from build123d import *

# Parameters (mm, degrees)
SKETCH_1_R      = 1.6
SKETCH_1_R_2    = 1.7
EXTRUDE_1_DEPTH = 3


with BuildPart() as part:
    # 草图1 → 凸台-拉伸1 (new body)
    with BuildSketch(Plane.XY):
        with BuildLine():
            Line((-53.850242828, 4), (171.149757172, 4))
            ThreePointArc((171.149757172, 4), (175.149757172, 0), (171.149757172, -4))
            Line((171.149757172, -4), (-53.850242828, -4))
            ThreePointArc((-53.850242828, -4), (-57.850242828, 0), (-53.850242828, 4))
        make_face()
        with Locations((-53.850242828, 0)):
            Circle(SKETCH_1_R, mode=Mode.SUBTRACT)
        with Locations((171.149757172, 0)):
            Circle(SKETCH_1_R_2, mode=Mode.SUBTRACT)
        with Locations((151.149757172, 0)):
            Circle(SKETCH_1_R_2, mode=Mode.SUBTRACT)
        with Locations((-33.850242828, 0)):
            Circle(SKETCH_1_R_2, mode=Mode.SUBTRACT)
    extrude(amount=EXTRUDE_1_DEPTH)


solid = part.part
For this review, take the finished solid that the model builds, in its own axes (mm). Give positions to 0.01 mm unless a question says otherwise; leave off trailing zeros. Order: outer loops, then holes, each group sorted by start corner. A loop starts at its lowest first (then second) coordinate and runs counter-clockwise, first axis right, second up. Notation, with made-up numbers: M -39,-2 L -15,-2 A27 ccw -15,16 Z; hole C -15.5,-14 d4. An arc over 180 degrees is marked long. Answer in a Markdown table with one row per item. Add a question column.
(1) Wall thickness on probe 1 along X at (y, z) = (1, 2.35); probe 2 along X at (y, z) = (1.25, 2.55); probe 3 along X at (y, z) = (3, 1.8): over which ranges is each line inside the solid? List them lowest first. Write a range as [from, to].
(2) Consider section A-A on y = 0. State the section outline as (x, z) points.
(3) For pin 1 (3 mm diameter, centred on x = 35.5, y = -2, fed in from -Z); pin 2 (2.5 mm diameter, centred on x = 171.15, y = 0, fed in from +Z), all flat-tipped, find the tip position at first contact; note any pin that passes through.
(4) Consider section B-B on z = 2.05. State the section outline as (x, y) points.
Evaluation:
| question | item | result |
|---|---|---|
| 1 | probe 1 | x = [-57.72, -55.1], [-52.6, -35.23], [-32.48, 149.77], [152.52, 169.77], [172.52, 175.02] |
| 1 | probe 2 | x = [-57.65, -54.85], [-52.85, -35], [-32.7, 150], [152.3, 170], [172.3, 174.95] |
| 1 | probe 3 | x = [-56.5, 173.8] |
| 2 | outline | M -57.85,0 L -55.45,0 L -55.45,3 L -57.85,3 Z; M -52.25,0 L -35.55,0 L -35.55,3 L -52.25,3 Z; M -32.15,0 L 149.45,0 L 149.45,3 L -32.15,3 Z; M 152.85,0 L 169.45,0 L 169.45,3 L 152.85,3 Z; M 172.85,0 L 175.15,0 L 175.15,3 L 172.85,3 Z |
| 3 | pin 1 | stops at z = 0 |
| 3 | pin 2 | passes through |
| 4 | outline | M -53.85,-4 L 171.15,-4 A4 ccw 171.15,4 L -53.85,4 A4 ccw Z; hole C -53.85,0 d3.2; hole C -33.85,0 d3.4; hole C 151.15,0 d3.4; hole C 171.15,0 d3.4 |
